```python
from build123d import *

# Parameters (mm, degrees)
SKETCH4_W           = 31.05
SKETCH4_H           = 18.55
BOSS_EXTRUDE1_DEPTH = 19
SHELL1_T            = 2
SKETCH5_W           = 12
SKETCH5_H           = 18.55
CUT_EXTRUDE1_DEPTH  = 2


with BuildPart() as part:
    # Sketch4 → Boss-Extrude1 (new body)
    with BuildSketch(Plane(origin=(0, 0, 0), x_dir=(0, 0, -1), z_dir=(1, 0, 0))):
        Rectangle(SKETCH4_W, SKETCH4_H)
    extrude(amount=BOSS_EXTRUDE1_DEPTH)

    # Shell1
    shell1_openings = [part.faces().sort_by_distance(p)[0] for p in [
        (0, 0, 0),
    ]]
    offset(amount=SHELL1_T, openings=shell1_openings, kind=Kind.INTERSECTION)

    # Sketch5 → Cut-Extrude1 (cut)
    with BuildSketch(Plane(origin=(0, 0, -17.525), x_dir=(-1, 0, 0), z_dir=(0, 0, -1))):
        with Locations((-6, 0)):
            Rectangle(SKETCH5_W, SKETCH5_H)
    extrude(amount=-CUT_EXTRUDE1_DEPTH, mode=Mode.SUBTRACT)


solid = part.part
```
Part model, mm, in its own coordinate system. A direction names the side the tool comes from. Round coordinates to 2 decimals unless told otherwise and drop trailing zeros. Write each loop counter-clockwise with the first axis right and the second up, starting at its lowest first coordinate (ties: lowest second). Pieces come first, ordered by that corner, then holes.
Item 1: Cut at C-C, the plane z = -8. Give the cut face in (x, y) (3 decimals).
Results:
outline: (0, -11.275) - (21, -11.275) - (21, 11.275) - (0, 11.275) - (0, 9.275) - (19, 9.275) - (19, -9.275) - (0, -9.275) - close
Item 2: Cut at B-B, the plane y = -5. Give the cut face in (x, z) (3 decimals), plus the area to 3 significant figures.
Results:
outline: (0, 15.525) - (19, 15.525) - (19, -15.525) - (12, -15.525) - (12, -17.525) - (21, -17.525) - (21, 17.525) - (0, 17.525) - close
area: 122 mm2
Item 3: Probe L1, parallel to Y at x = 16.5, z = -1.5 (3 decimals); L2, parallel to Z at x = 14.5, y = -2.75 (3 decimals); L3, parallel to X at y = -5.75, z = -1. List the from-to ranges inside material, lowest first.
Results:
L1: y = -11.275 to -9.275, 9.275 to 11.275
L2: z = -17.525 to -15.525, 15.525 to 17.525
L3: x = 19 to 21
Item 4: Drop a flat-ended pin along its axis: pin 1 Ø0.6 at (y, z) = (4.5, -16.5) entering from -X. Give the stop position or say it passes through.
Results:
pin 1: stops at x = 12
Item 5: Which spindle directions (+Z, -Z, +X, -X, +Y, -Y) get a long thin tool onto all of the face, cutting with end or side? Do faces 1 (the flat face through (12, 0, -17)), 2 (the flat face through (15, 0, -15.525)), 3 (the flat face through (21, 0, 0)). Say none if no direction does.
Results:
face 1: -Z, -X
face 2: -X
face 3: +Z, -Z, +X, +Y, -Y
Item 6: Two-plate mould, pull along Y, no slides. Class faces 4 (the flat face through (9, 9.275, -1)), 5 (the flat face through (10, 11.275, 0)), 6 (the flat face through (0, -10, 4)): +Y half, -Y half, draft (parallel to the pull), parting line (faces both ways), or undercut.
Results:
face 4: undercut
face 5: +Y half
face 6: draft
Item 7: Cut at A-A, the plane x = 18.5. Give the cut face in (y, z) (3 decimals).
Results:
outline: (-11.275, -17.525) - (11.275, -17.525) - (11.275, 17.525) - (-11.275, 17.525) - close; hole (-9.275, -15.525) - (9.275, -15.525) - (9.275, 15.525) - (-9.275, 15.525) - close
